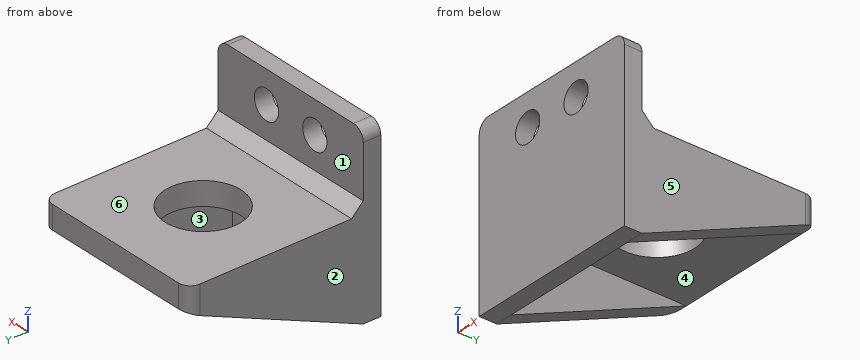
Autodesk Inventor part; units mm, degrees
ref_plane "Work Plane1" through (0, 15, 4) normal (1, 0, 0) x (0, 0, -1)
ref_plane "YZ Plane" through (0, 0, 0) normal (1, 0, 0) x (0, 1, 0)
ref_plane "XZ Plane" through (0, 0, 0) normal (0, 1, 0) x (-1, 0, 0)
sketch "Sketch1" plane through (0, 0, 0) normal (0, 0, 1) x (1, 0, 0)
  line L0 (-15, 15) -> (15, 15)
  line L1 (15, 15) -> (15, -15)
  line L2 (15, -15) -> (-15, -15)
  line L3 (-15, -15) -> (-15, 15)
  line L4 (-15, 15) -> (15, -15) construction
  line L5 (15, 15) -> (-15, -15) construction
  circle A0 centre (0, 0) radius 6.5
  dimension "d0" = 30
  dimension "d1" = 30
  dimension "d2" = 13
extrude "Extrusion1" add sketch "Sketch1" along normal blind 4
sketch "Sketch2" plane through (-15, -15, 0) normal (0, -1, 0) x (1, 0, 0)
  line L0 (0, 17) -> (30, 17)
  line L1 (30, 17) -> (30, -13)
  line L2 (30, -13) -> (0, -13)
  line L3 (0, -13) -> (0, 17)
  line L4 (0, 17) -> (30, -13) construction
  line L5 (30, 17) -> (0, -13) construction
  point P0 (15, 0)
  point P1 (15, 2)
  dimension "d5" = 30
  dimension "d6" = 30
extrude "Extrusion2" add sketch "Sketch2" along normal blind 3
ref_plane "Work Plane1" through (0, 15, 4) normal (1, 0, 0) x (0, 0, -1)
sketch "Sketch3" plane through (15, 15, 4) normal (1, 0, 0) x (0, 0, -1)
  line L0 (-13, -33) -> (17, -33)
  line L1 (0.0291, -33) -> (0.0291, 0)
  line L2 (4, 0) -> (4, -30)
  line L3 (0.0291, 0) -> (4, 0)
  line L4 (4, -30) -> (17, -30)
  line L5 (4, 0) -> (17, -30)
  line L6 (17, -30) -> (17, -33)
  line L7 (17, -30) -> (17, -33)
  line L8 (17, -33) -> (0.0291, -33)
  point P0 (4, -15)
extrude "Extrusion3" add sketch "Sketch3" against normal blind 3 contours L4 L2 L5
mirror "Mirror1" about plane through (0, 15, 4) normal (1, 0, 0) of "Extrusion3"
chamfer "Chamfer1" distance 2 angle 45 1 edges at (0, -15, 4)
sketch "Sketch4" plane through (-15, -15, 0) normal (0, 1, 0) x (1, 0, 0)
  line L0 (0, -17) -> (30, -17)
  line L1 (0, -6) -> (0, -17)
  point P0 (15, 0)
  point P1 (10, -11.5)
  point P2 (20, -11.5)
  dimension "d15" = 5.5
  dimension "d16" = 10
  dimension "d25" = 5.5
  dimension "d26" = 20
hole "Hole1" at (-5, -15, 11.5) at (5, -15, 11.5) direction (0, -1, 0) diameter 5 end through all
fillet "Fillet1" radius 2 4 edges at (-15, 15, 2) (15, 15, 2) (15, -16.5, 17) (-15, -16.5, 17)
properties part number "Eletronica - plug12V"
Check sheet for the modelled part. Datum: model origin and axes. Units: mm. Face numbers are marked on the shaded views. A direction names the side the tool comes from. Round coordinates to 2 decimals unless told otherwise and drop trailing zeros. Write each loop counter-clockwise with the first axis right and the second up, starting at its lowest first coordinate (ties: lowest second). Pieces come first, ordered by that corner, then holes. Notation, with made-up numbers: M 14,70 L 56,70 A24 ccw 56,80 Z; hole C 3,-24.75 d6. An arc over 180 degrees is marked long. Write item = value, one per line. Start each with the question number.
1. Section check A-A, the plane y = 0. Record the cut outline in (x, z), then the cut area to 3 significant figures.
2. Tool access check on the marked faces 1, 2 and 3. Record the directions out of +Z, -Z, +X, -X, +Y, -Y that give a thin tool (end or side, any length) a straight path to the whole face; none if there is none.
3. Section check D-D, the plane x = 3.5. Record the cut outline in (y, z), then the cut area to 3 significant figures.
4. Scan lines: line 1 (X direction, y = -15.75, z = 11.5); line 2 (X direction, y = -6.5, z = -3); line 3 (Z direction, x = -5, y = -16.3). Record each from-to range of solid material in increasing order. Write a range as [from, to].
5. Section check C-C, the plane z = 11.5. Record the cut outline in (x, y), then the cut area to 3 significant figures.
6. Release check for a two-part mould opening along X. For the marked faces 4, 5 and 6 record: pulls with the +X half, pulls with the -X half, needs draft (parallel to the pull), parting line crosses it, or undercut.
7. Gauge pin test, flat ends, axial feed: pin 1 (2 mm diameter, centred on x = -4.5, z = 5.5, fed in from +Y); pin 2 (1 mm diameter, centred on x = -1, z = 9.5, fed in from +Y); pin 3 (6 mm diameter, centred on x = -3, y = -2, fed in from +Z); pin 4 (4 mm diameter, centred on x = 5, z = 11.5, fed in from +Y). Record the tip position at first contact, or that the pin passes through.
8. Section check B-B, the plane x = 0. Record the cut outline in (y, z).
Results found:
q1.outline = M -15,-6.5 L -12,-6.5 L -12,0 L -6.5,0 L -6.5,4 L -15,4 Z; M 6.5,0 L 12,0 L 12,-6.5 L 15,-6.5 L 15,4 L 6.5,4 Z
q1.area = 107 mm^2
q2.face_1 = +Z, +X, -X, +Y
q2.face_2 = +Z, -Z, -X, +Y, -Y
q2.face_3 = -Z, +Y
q3.outline = M -18,-13 L -15,-13 L -15,0 L -5.48,0 L -5.48,4 L -13,4 L -15,6 L -15,9.5 L -18,9.5 Z; M -18,13.5 L -15,13.5 L -15,17 L -18,17 Z; M 5.48,0 L 15,0 L 15,4 L 5.48,4 Z
q3.area = 156 mm^2
q4.line_1 = [-15, -7.5], [-2.5, 2.5], [7.5, 15]
q4.line_2 = [-15, -12], [12, 15]
q4.line_3 = [-13, 9], [14, 17]
q5.outline = M -15,-18 L -7.5,-18 L -7.5,-15 L -15,-15 Z; M -2.5,-18 L 2.5,-18 L 2.5,-15 L -2.5,-15 Z; M 7.5,-18 L 15,-18 L 15,-15 L 7.5,-15 Z
q5.area = 60.0 mm^2
q6.face_4 = undercut
q6.face_5 = pulls with the +X half
q6.face_6 = needs draft
q7.pin_1 = -13.5
q7.pin_2 = -15
q7.pin_3 = 4
q7.pin_4 = through
q8.outline = M -18,-13 L -15,-13 L -15,0 L -6.5,0 L -6.5,4 L -13,4 L -15,6 L -15,17 L -18,17 Z; M 6.5,0 L 15,0 L 15,4 L 6.5,4 Z
